```python
from build123d import *

# Parameters (mm, degrees)
BOSS_EXTRUDE1_DEPTH                                  = 5
BOSS_EXTRUDE1_DEPTH_BACK                             = 5
SKETCH1_W                                            = 200
SKETCH1_H                                            = 200
TAP_DRILL_FOR_M5X0_8_TAP1_D                          = 5
SKETCH5_W                                            = 50
SKETCH5_H                                            = 25
CUT_EXTRUDE2_DEPTH                                   = 20
CBORE_FOR_M6_PAN_HEAD_SCREW1_D                       = 6.6
CBORE_FOR_M6_PAN_HEAD_SCREW1_CBORE_D                 = 13
CBORE_FOR_M6_PAN_HEAD_SCREW1_CBORE_DEPTH             = 4.6
CSK_FOR_M5_HEX_SOCKET_COUNTERSUNK_CAP_SC_D           = 5.5
CSK_FOR_M5_HEX_SOCKET_COUNTERSUNK_CAP_SC_CSINK_D     = 11.2
CSK_FOR_M5_HEX_SOCKET_COUNTERSUNK_CAP_SC_CSINK_ANGLE = 90


with BuildPart() as part:
    # Sketch1 → Boss-Extrude1 (new, two sides: drawn at the far end of the back side and taken through both)
    with BuildSketch(Plane.XY.offset(-BOSS_EXTRUDE1_DEPTH_BACK)):
        Rectangle(SKETCH1_W, SKETCH1_H)
    extrude(amount=BOSS_EXTRUDE1_DEPTH + BOSS_EXTRUDE1_DEPTH_BACK)

    # Tap Drill for M5x0.8 Tap1 (through all)
    with Locations(Plane(origin=(0, 0, -5), x_dir=(-1, 0, 0), z_dir=(0, 0, -1))):
        with Locations((-52, 57), (52, 57), (52, -57), (-52, -57)):
            Hole(TAP_DRILL_FOR_M5X0_8_TAP1_D / 2)

    # Sketch5 → Cut-Extrude2 (cut)
    with BuildSketch(Plane(origin=(0, 0, -5), x_dir=(-1, 0, 0), z_dir=(0, 0, -1))):
        Rectangle(SKETCH5_W, SKETCH5_H)
    extrude(amount=-CUT_EXTRUDE2_DEPTH, mode=Mode.SUBTRACT)

    # CBORE for M6 Pan Head Screw1 (through all)
    with Locations(Plane.XY.offset(5)):
        with Locations((-80, 80), (-80, 0), (-80, -80), (80, 80), (80, 0), (80, -80), (0, 80), (0, -80)):
            CounterBoreHole(CBORE_FOR_M6_PAN_HEAD_SCREW1_D / 2, CBORE_FOR_M6_PAN_HEAD_SCREW1_CBORE_D / 2, CBORE_FOR_M6_PAN_HEAD_SCREW1_CBORE_DEPTH)

    # CSK for M5 Hex Socket Countersunk Cap Screw1 (through all)
    with Locations(Plane(origin=(0, 0, -5), x_dir=(-1, 0, 0), z_dir=(0, 0, -1))):
        with Locations((-52, 57), (52, 57), (52, -57), (-52, -57)):
            CounterSinkHole(CSK_FOR_M5_HEX_SOCKET_COUNTERSUNK_CAP_SC_D / 2, CSK_FOR_M5_HEX_SOCKET_COUNTERSUNK_CAP_SC_CSINK_D / 2, counter_sink_angle=CSK_FOR_M5_HEX_SOCKET_COUNTERSUNK_CAP_SC_CSINK_ANGLE)


solid = part.part
```
Source: CAD feature listing. Evaluate the final solid. Frame: model axes, mm. A direction names the side the tool comes from. Round coordinates to 2 decimals unless told otherwise and drop trailing zeros. Order: outer loops, then holes, each group sorted by start corner. A loop starts at its lowest first (then second) coordinate and runs counter-clockwise, first axis right, second up. Notation, with made-up numbers: (-7.5, 66) -> (47.5, 66) arc R19 cw to (47.5, 81) -> close; hole circle Ø4 at (41, -25). An arc over 180 degrees is marked (long way). One line per item, written item: value. Start each with the question number.
Q1. Access query for faces 4 (the flat face through (-3, -78, 0.4)), 5 (the conical face through (54.755, 57.868, -2.288)), 6 (the flat face through (-25, 0, 0)). Directions: +Z, -Z, +X, -X, +Y, -Y. A direction counts if a zero-diameter tool reaches every point of the face in a straight line with its end or side. Return the directions, or none.
Q2. Draft query along Y for faces 1 (the flat face through (77, -78, 0.4)), 2 (the flat face through (-1, 100, 0)), 3 (the flat face through (-1, -100, 0)). Return one class per face: pulls with the +Y half, pulls with the -Y half, needs draft (parallel to the pull), parting line crosses it, or undercut.
Q3. Section query B-B (z = 3.5). Give the number of separate pieces and of enclosed holes in the cut face, plus the area to 3 significant figures.
Q4. Section query C-C (x = 52). Return the cut outline in (y, z).
Q5. Section query A-A (x = -80). Return the cut outline in (y, z).
Q6. Pin query (flat end, axial travel): pin 1 (8 mm diameter, centred on x = 80, y = -80, fed in from +Z); pin 2 (7 mm diameter, centred on x = -52, y = 57, fed in from -Z); pin 3 (4 mm diameter, centred on x = -80, y = -80, fed in from +Z); pin 4 (6.5 mm diameter, centred on x = -77, y = -2.5, fed in from +Z). Return the tip coordinate at first contact, or that it passes through.
Q7. Material intervals for probe 1 along Y at (x, z) = (-52, 1.25); probe 2 along Y at (x, z) = (80, 2.7); probe 3 along Y at (x, z) = (80, -3.75), sorted ascending.
Findings below:
1. face 4: +Z
1. face 5: -Z
1. face 6: +Z, -Z
2. face 1: undercut
2. face 2: pulls with the +Y half
2. face 3: pulls with the -Y half
3. separate pieces: 1
3. enclosed holes: 13
3. area: 37,600 mm²
4. outline: (-100, -5) -> (-62.6, -5) -> (-59.75, -2.15) -> (-59.75, 5) -> (-100, 5) -> close; (-54.25, -2.15) -> (-51.4, -5) -> (51.4, -5) -> (54.25, -2.15) -> (54.25, 5) -> (-54.25, 5) -> close; (59.75, -2.15) -> (62.6, -5) -> (100, -5) -> (100, 5) -> (59.75, 5) -> close
5. outline: (-100, -5) -> (-83.3, -5) -> (-83.3, 0.4) -> (-86.5, 0.4) -> (-86.5, 5) -> (-100, 5) -> close; (-76.7, -5) -> (-3.3, -5) -> (-3.3, 0.4) -> (-6.5, 0.4) -> (-6.5, 5) -> (-73.5, 5) -> (-73.5, 0.4) -> (-76.7, 0.4) -> close; (3.3, -5) -> (76.7, -5) -> (76.7, 0.4) -> (73.5, 0.4) -> (73.5, 5) -> (6.5, 5) -> (6.5, 0.4) -> (3.3, 0.4) -> close; (83.3, -5) -> (100, -5) -> (100, 5) -> (86.5, 5) -> (86.5, 0.4) -> (83.3, 0.4) -> close
6. pin 1: z = 0.4
6. pin 2: z = -2.9
6. pin 3: through
6. pin 4: z = 5
7. probe 1: -100 to -59.75, -54.25 to 54.25, 59.75 to 100
7. probe 2: -100 to -86.5, -73.5 to -6.5, 6.5 to 73.5, 86.5 to 100
7. probe 3: -100 to -83.3, -76.7 to -3.3, 3.3 to 76.7, 83.3 to 100
